Job drawing, mm, ordinate dimensions from the low corner. One solid piece. A direction names the side the tool comes from. Give positions to 0.01 mm unless a question says otherwise; leave off trailing zeros. Write each loop counter-clockwise with the first axis right and the second up, starting at its lowest first coordinate (ties: lowest second). Pieces come first, ordered by that corner, then holes. Notation, with made-up numbers: M 26.5,10.25 L 44.5,10.25 A19 cw 44.5,34.25 Z; hole C -7,34 d3. An arc over 180 degrees is marked long. Use a Markdown table: item, result.
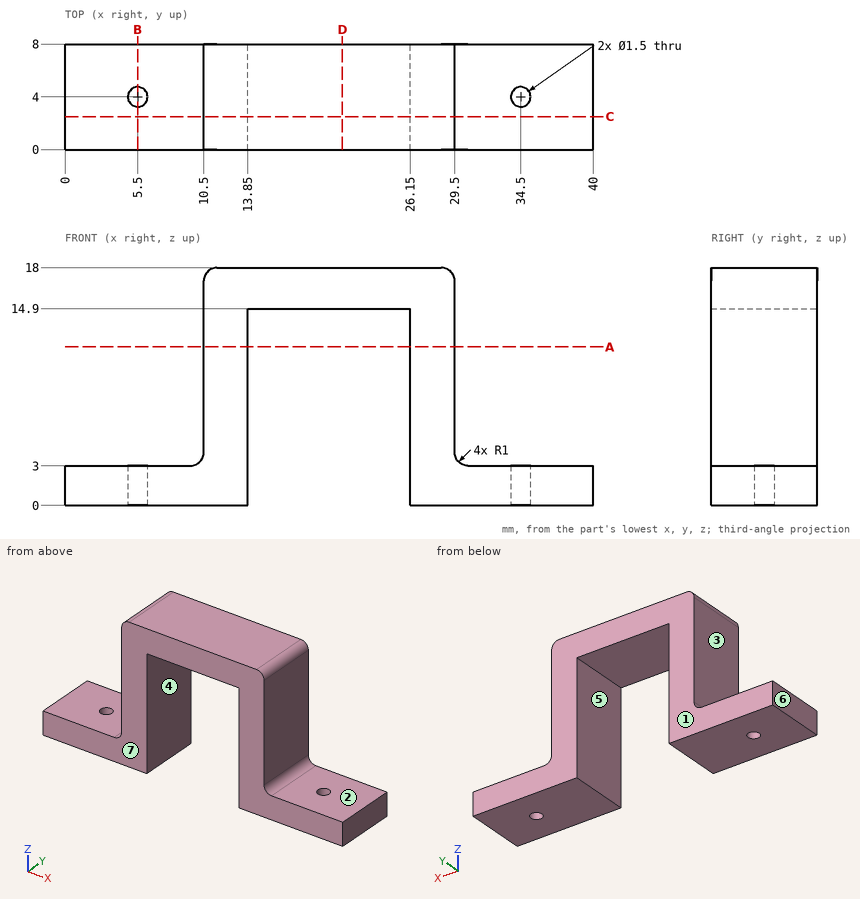
1. Tool access for the marked faces 1, 2, 3 and 4: list every direction of +Z, -Z, +X, -X, +Y, -Y with a clear straight run to the whole face (end or side of a thin tool).
Findings below:
| item | result |
|---|---|
| face 1 | +Z, -Z, +X, -X, +Y |
| face 2 | +Z, +X, +Y, -Y |
| face 3 | +Z, -X, +Y, -Y |
| face 4 | -Z, +Y, -Y |
2. Cut at B-B, the plane x = 5.5. Give the cut face in (y, z).
Findings below:
| item | result |
|---|---|
| outline | M 0,0 L 3.25,0 L 3.25,3 L 0,3 Z; M 4.75,0 L 8,0 L 8,3 L 4.75,3 Z |
3. Drill centre lines: L1, parallel to X at y = 1.5, z = 4.5; L2, parallel to Y at x = 34.5, z = 1.7; L3, parallel to X at y = 5, z = 2. Where is each one in solid material? Low to high.
Findings below:
| item | result |
|---|---|
| L1 | 10.5 to 13.85, 26.15 to 29.5 |
| L2 | 0 to 3.25, 4.75 to 8 |
| L3 | 0 to 13.85, 26.15 to 40 |
4. Cut at D-D, the plane x = 21. Give the cut face in (y, z).
Findings below:
| item | result |
|---|---|
| outline | M 0,14.9 L 8,14.9 L 8,18 L 0,18 Z |
5. Cut at C-C, the plane y = 2.5. Give the cut face in (x, z).
Findings below:
| item | result |
|---|---|
| outline | M 0,0 L 13.85,0 L 13.85,14.9 L 26.15,14.9 L 26.15,0 L 40,0 L 40,3 L 30.5,3 A1 cw 29.5,4 L 29.5,17 A1 ccw 28.5,18 L 11.5,18 A1 ccw 10.5,17 L 10.5,4 A1 cw 9.5,3 L 0,3 Z |
6. Cut at A-A, the plane z = 12. Give the cut face in (x, y).
Findings below:
| item | result |
|---|---|
| outline | M 10.5,0 L 13.85,0 L 13.85,8 L 10.5,8 Z; M 26.15,0 L 29.5,0 L 29.5,8 L 26.15,8 Z |
7. Drop flat-ended pins along their axis: P1, Ø1, axis at y = 2.5, z = 14, coming from the -X side; P2, Ø6, axis at x = 7, z = 10.5, coming from the -Y side. Give the stop position or say it passes through.
Findings below:
| item | result |
|---|---|
| P1 | x = 10.5 |
| P2 | through |
8. Two-plate mould, pull along X, no slides. Class the marked faces 5, 6 and 7: released by +X, released by -X, zero draft, split by the parting line, or undercut.
Findings below:
| item | result |
|---|---|
| face 5 | undercut |
| face 6 | released by -X |
| face 7 | zero draft |
